Print and shaded views of the part. All mm, measured from the part's lowest x, y and z. Coordinates: 2 decimals unless noted, no trailing zeros. Order: outer loops, then holes, each group sorted by start corner. A loop starts at its lowest first (then second) coordinate and runs counter-clockwise, first axis right, second up. Notation, with made-up numbers: (80.5, 37.25) -> (91.5, 37.25) arc R28 ccw to (91.5, 62.25) -> close; hole circle Ø5 at (-22, -24.75). An arc over 180 degrees is marked (long way). Write item = value, one per line. Start each with the question number.
Q1. Wall check: line 1 (X direction, y = 7.55, z = 37.7); line 2 (Y direction, x = 29, z = 8.5); line 3 (X direction, y = 7.75, z = 40). Give the ranges that are in metal, low to high. Write a range as from..to.
Q2. Cut at A-A, the plane z = 37.7. List the corners of the cut face in (x, y), plus the area to 3 significant figures.
Q3. Cut at D-D, the plane z = 46.5. List the corners of the cut face in (x, y).
Q4. Cut at B-B, the plane x = 37.7. List the corners of the cut face in (y, z).
Q5. Cut at C-C, the plane x = 28. List the corners of the cut face in (y, z), plus the area to 3 significant figures.
Q6. Mould opens along Z. For the marked faces 1 and 2 say: +Z half, -Z half, draft (parallel to the pull), parting line (faces both ways), or undercut.
Q7. Flat gauge pins, fed straight in: pin 1 (2.5 mm diameter, centred on x = 12.3, z = 37.7, fed in from +Y); pin 2 (2 mm diameter, centred on x = 43, y = 7, fed in from -Z). Where does each tip first touch, or does it go through?
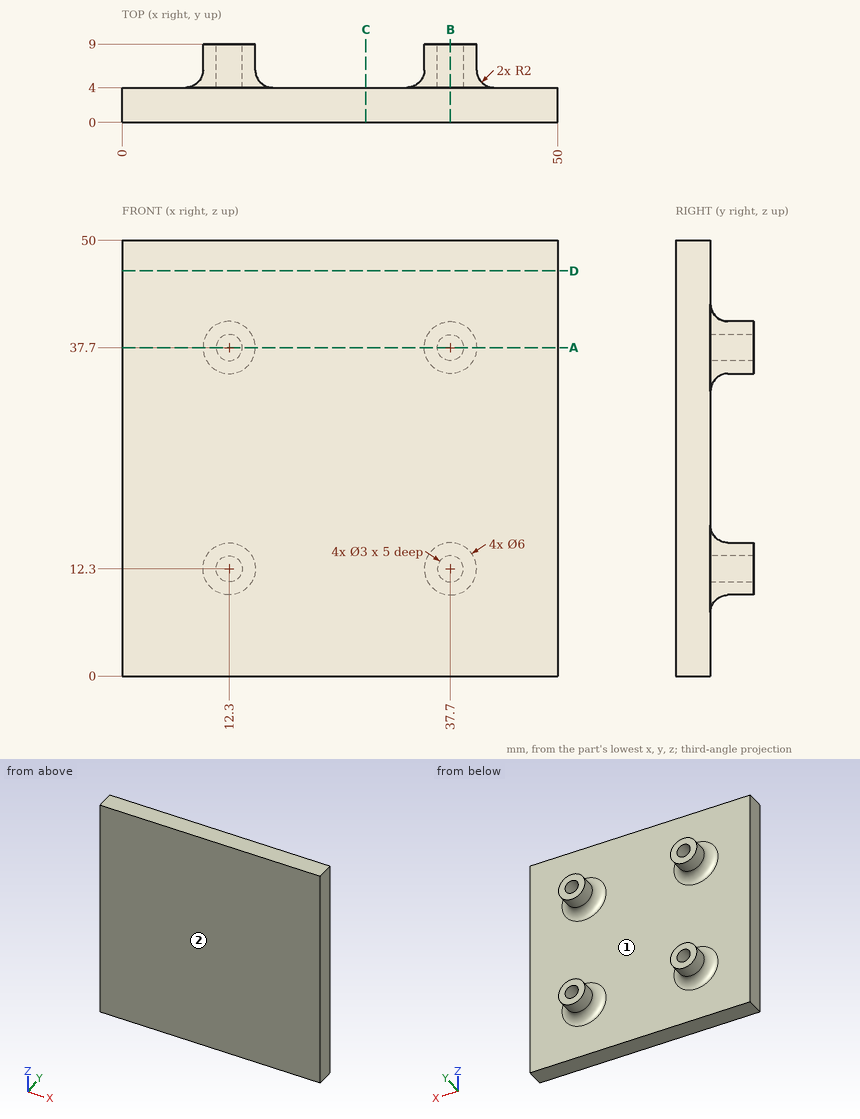
Here are the results:
q1.line_1 = 9.3..10.8, 13.8..15.3, 34.7..36.2, 39.2..40.7
q1.line_2 = 0..4
q1.line_3 = 10.37..14.23, 35.77..39.63
q2.outline = (0, 0) -> (50, 0) -> (50, 4) -> (42.7, 4) arc R2 cw to (40.7, 6) -> (40.7, 9) -> (39.2, 9) -> (39.2, 4) -> (36.2, 4) -> (36.2, 9) -> (34.7, 9) -> (34.7, 6) arc R2 cw to (32.7, 4) -> (17.3, 4) arc R2 cw to (15.3, 6) -> (15.3, 9) -> (13.8, 9) -> (13.8, 4) -> (10.8, 4) -> (10.8, 9) -> (9.3, 9) -> (9.3, 6) arc R2 cw to (7.3, 4) -> (0, 4) -> close
q2.area = 233 mm²
q3.outline = (0, 0) -> (50, 0) -> (50, 4) -> (0, 4) -> close
q4.outline = (0, 0) -> (4, 0) -> (4, 7.3) arc R2 cw to (6, 9.3) -> (9, 9.3) -> (9, 10.8) -> (4, 10.8) -> (4, 13.8) -> (9, 13.8) -> (9, 15.3) -> (6, 15.3) arc R2 cw to (4, 17.3) -> (4, 32.7) arc R2 cw to (6, 34.7) -> (9, 34.7) -> (9, 36.2) -> (4, 36.2) -> (4, 39.2) -> (9, 39.2) -> (9, 40.7) -> (6, 40.7) arc R2 cw to (4, 42.7) -> (4, 50) -> (0, 50) -> close
q5.outline = (0, 0) -> (4, 0) -> (4, 50) -> (0, 50) -> close
q5.area = 200 mm²
q6.face_1 = undercut
q6.face_2 = draft
q7.pin_1 = 4
q7.pin_2 = through
